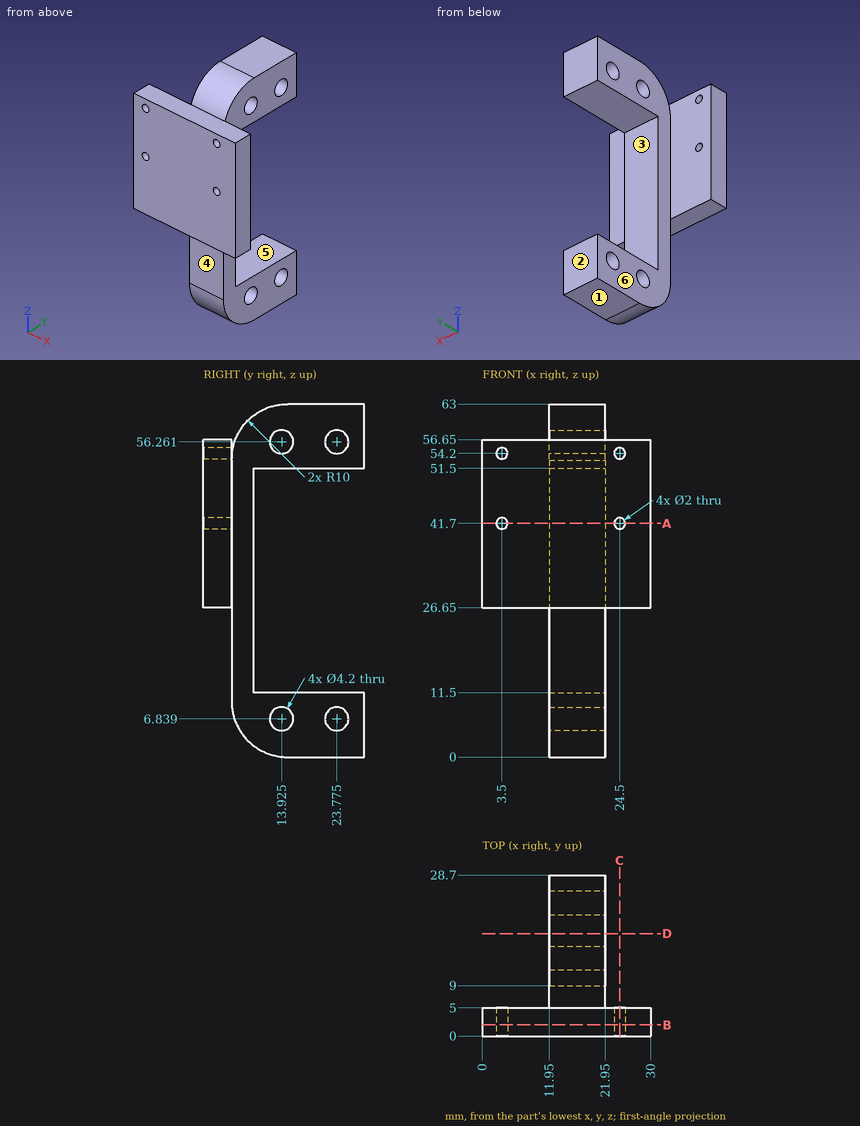
The figure shows three views and two pictorial views of one solid part (mm, origin at its lowest corner). Answer the questions. A direction names the side the tool comes from. Coordinates: 2 decimals unless noted, no trailing zeros. Loops run counter-clockwise (first coordinate to the right, second up) from the corner with the lowest first, then second, coordinate; pieces in that order, holes last. Notation, with made-up numbers: (46.5, 3.5) - (51.5, 3.5) arc R19 ccw to (51.5, 12.5) - close; hole circle Ø1 at (-9.75, -37). An arc over 180 degrees is marked (long way). Answer in a Markdown table with one row per item.
Q1. Find section C-C on x = 24.5. Write down the section's boundary in (y, z).
Here are the results:
| item | result |
|---|---|
| outline | (0, 26.65) - (5, 26.65) - (5, 40.7) - (0, 40.7) - close; (0, 42.7) - (5, 42.7) - (5, 53.2) - (0, 53.2) - close; (0, 55.2) - (5, 55.2) - (5, 56.65) - (0, 56.65) - close |
Q2. The mould has two halves that part along Z. Classify the marked faces 1, 2 and 3: pulls with the +Z half, pulls with the -Z half, needs draft (parallel to the pull), parting line crosses it, or undercut.
Here are the results:
| item | result |
|---|---|
| face 1 | pulls with the -Z half |
| face 2 | needs draft |
| face 3 | undercut |
Q3. Find section D-D on y = 18.25. Write down the section's boundary in (x, z), plus the area to 3 significant figures.
Here are the results:
| item | result |
|---|---|
| outline | (11.95, 0) - (21.95, 0) - (21.95, 11.5) - (11.95, 11.5) - close; (11.95, 51.5) - (21.95, 51.5) - (21.95, 63) - (11.95, 63) - close |
| area | 230 mm^2 |
Q4. Find section B-B on y = 2. Write down the section's boundary in (x, z), plus the area to 3 significant figures.
Here are the results:
| item | result |
|---|---|
| outline | (0, 26.65) - (30, 26.65) - (30, 56.65) - (0, 56.65) - close; hole circle Ø2 at (3.5, 41.7); hole circle Ø2 at (3.5, 54.2); hole circle Ø2 at (24.5, 41.7); hole circle Ø2 at (24.5, 54.2) |
| area | 887 mm^2 |
Q5. Straight lines are drawn through the part: line 1 along X through (y, z) = (2.8, 41.7); line 2 along Z through (x, y) = (13.75, 18); line 3 along Y through (x, z) = (17.75, 55). For each, find the intervals that lie inside material, in ascending order. Write a range as [from, to].
Here are the results:
| item | result |
|---|---|
| line 1 | x = [0, 2.5], [4.5, 23.5], [25.5, 30] |
| line 2 | z = [0, 11.5], [51.5, 63] |
| line 3 | y = [0, 5], [5.2, 12.25], [15.6, 22.1], [25.45, 28.7] |
Q6. Given P1, Ø8, axis at x = 13, z = 17, coming from the -Y side; P2, Ø5, axis at y = 13.92, z = 56.26, coming from the -X side; P3, Ø6.5, axis at y = 13.92, z = 6.84, coming from the +X side; P4, Ø6, axis at x = 27, y = 11, coming from the -Z side, each flat-ended and moving along its own axis, determine where each tip first touches the part or whether it passes through.
Here are the results:
| item | result |
|---|---|
| P1 | stops at y = 5 |
| P2 | stops at x = 11.95 |
| P3 | stops at x = 21.95 |
| P4 | passes through |
Q7. Find section A-A on z = 41.7. Write down the section's boundary in (x, y).
Here are the results:
| item | result |
|---|---|
| outline | (0, 0) - (2.5, 0) - (2.5, 5) - (0, 5) - close; (4.5, 0) - (23.5, 0) - (23.5, 5) - (21.95, 5) - (21.95, 9) - (11.95, 9) - (11.95, 5) - (4.5, 5) - close; (25.5, 0) - (30, 0) - (30, 5) - (25.5, 5) - close |
Q8. For the marked faces 4, 5 and 6, determine the directions among +Z, -Z, +X, -X, +Y, -Y from which every point of the face is accessible in a straight line to the end or side of a thin tool.
Here are the results:
| item | result |
|---|---|
| face 4 | -Z, +X, -X, -Y |
| face 5 | +X, -X, +Y |
| face 6 | +Z, -Z, -X, +Y |
